```python
from build123d import *

# Parameters (mm, degrees)
F0_R     = 9
F1_DEPTH = 20
F1_TAPER = 5
F2_R     = 7.5
F2_R_2   = 7.2502267295
F3_DEPTH = 10
F4_R     = 9
F4_R_2   = 7.5
F5_DEPTH = 8
F7_DEPTH = 14


with BuildPart() as f1:
    # F0 (on Top) → F1 (new body)
    with BuildSketch(Plane.XY):
        Circle(F0_R)
    extrude(amount=F1_DEPTH, taper=F1_TAPER)

    # F2 (on face) → F3 (join)
    with BuildSketch(Plane.XY.offset(20)):
        Circle(F2_R)
        Circle(F2_R_2, mode=Mode.SUBTRACT)
    extrude(amount=-F3_DEPTH)

    # F4 (on face) → F5 (cut)
    with BuildSketch(Plane.XY.offset(20)):
        Circle(F4_R)
        Circle(F4_R_2, mode=Mode.SUBTRACT)
    extrude(amount=-F5_DEPTH, mode=Mode.SUBTRACT)

    # F6 (on face) → F7 (cut)
    with BuildSketch(Plane.XY.offset(20)):
        with BuildLine():
            Line((6.8738635424, -3), (8.9953789802, -3))
            Line((8.9953789802, -3), (8.9953789802, 3))
            Line((8.9953789802, 3), (6.8738635424, 3))
            ThreePointArc((6.8738635424, 3), (7.341797347, 1.5323223277), (7.5, 0))
            ThreePointArc((7.5, 0), (7.341797347, -1.5323223277), (6.8738635424, -3))
        make_face()
        with BuildLine():
            Line((3, -3), (6.8738635424, -3))
            ThreePointArc((6.8738635424, -3), (7.341797347, -1.5323223277), (7.5, 0))
            ThreePointArc((7.5, 0), (7.341797347, 1.5323223277), (6.8738635424, 3))
            Line((6.8738635424, 3), (3, 3))
            Line((3, 3), (3, -3))
        make_face()
    extrude(amount=-F7_DEPTH, mode=Mode.SUBTRACT)


solid = f1.part
```
Can you work these out from the model? Positions are in its coordinate system, mm. A direction names the side the tool comes from. Round coordinates to 2 decimals unless told otherwise and drop trailing zeros. Loops run counter-clockwise (first coordinate to the right, second up) from the corner with the lowest first, then second, coordinate; pieces in that order, holes last.
Item 1: Which directions (+Z, -Z, +X, -X, +Y, -Y) give clear straight access to the entire face, cutting with the end or side of a thin tool? Please do faces 1 (the flat face through (0, 0, 20)), 2 (the cylindrical face through (-7.495, 0.287, 16.056)), 3 (the flat face through (6, 0, 6)).
Item 2: If we mould it in two halves opening along Y, with no side actions, what happens to faces 4 (the flat face through (5, 3, 13)), 5 (the flat face through (-7.7, 0, 12)), 6 (the conical face through (-6.72, -5.15, 6.08))? For each: +Y half, -Y half, draft (parallel to the pull), parting line (faces both ways), or undercut.
Item 3: Suppose I cut it at C-C, the plane z = 5.5. Write out the boundary of the cut face in (x, y), then the cut area to 3 significant figures.
Item 4: Suppose I cut it at A-A, the plane x = 0. Write out the boundary of the cut face in (y, z).
Item 5: Suppose I cut it at D-D, the plane z = 2.5. Write out the boundary of the cut face in (x, y), then the cut area to 3 significant figures.
Item 6: Will these pins go through, and if not, where does the flat tip stop? pin 1 Ø8 at (y, z) = (0, 6) entering from -X (3 decimals); pin 2 Ø1.5 at (y, z) = (6, 17) entering from +X; pin 3 Ø4 at (x, z) = (6, 11.5) entering from -Y; pin 4 Ø4.5 at (x, y) = (5.5, 1.5) entering from +Z.
Item 7: Suppose I cut it at B-B, the plane y = 0. Write out the boundary of the cut face in (x, z), then the cut area to 3 significant figures.
Item 8: Please list where these lines run through material, in increasing order: L1, parallel to Z at x = 8, y = 0.5; L2, parallel to Y at x = 5.5, z = 9.5; L3, parallel to Y at x = 7, z = 6.5.
Reported:
1. face 1: +Z, +X, -X, +Y, -Y
1. face 2: +Z
1. face 3: +Z, +X
2. face 4: undercut
2. face 5: draft
2. face 6: parting line
3. outline: circle Ø17.04 at (0, 0)
3. area: 228 mm2
4. outline: (-9, 0) - (9, 0) - (7.95, 12) - (7.5, 12) - (7.5, 20) - (-7.5, 20) - (-7.5, 12) - (-7.95, 12) - close
5. outline: circle Ø17.56 at (0, 0)
5. area: 242 mm2
6. pin 1: stops at x = -8.825
6. pin 2: stops at x = 5.36
6. pin 3: stops at y = -6.94
6. pin 4: stops at z = 20
7. outline: (-9, 0) - (9, 0) - (8.48, 6) - (3, 6) - (3, 20) - (-7.5, 20) - (-7.5, 12) - (-7.95, 12) - close
7. area: 256 mm2
8. L1: z = 0 to 6
8. L2: y = -6.04 to -3, 3 to 6.04
8. L3: y = -4.7 to -3, 3 to 4.7
